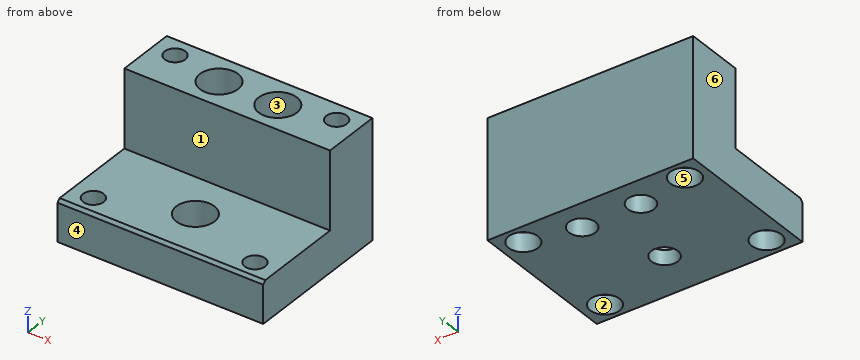
```python
from build123d import *

# Parameters (mm, degrees)
SKIZZE1_W                                            = 140
SKIZZE1_H                                            = 103
BASIS_LINEAR_AUSTRAGEN_DEPTH                         = 40.5
SKIZZE8_W                                            = 53
SKIZZE8_H                                            = 63
SCHNITT_LINEAR_AUSTRAGEN1_DEPTH                      = 155.571989701
BOHRUNG1_D                                           = 18
BOHRUNG1_DEPTH                                       = 90
BOHRUNG1_CBORE_D                                     = 26
BOHRUNG1_CBORE_DEPTH                                 = 18
BOHRUNG2_D                                           = 18
BOHRUNG2_DEPTH                                       = 90
BOHRUNG2_CBORE_D                                     = 26
BOHRUNG2_CBORE_DEPTH                                 = 18
LINEARES_MUSTER1_COUNT                               = 2
LINEARES_MUSTER1_PITCH                               = 40
STIRNSENKUNG_F_R_M8_FLACHKOPFSCHRAUBE_MI_D           = 14
STIRNSENKUNG_F_R_M8_FLACHKOPFSCHRAUBE_MI_CBORE_D     = 20
STIRNSENKUNG_F_R_M8_FLACHKOPFSCHRAUBE_MI_CBORE_DEPTH = 13
SKIZZE11_R                                           = 13
SCHNITT_LINEAR_AUSTRAGEN2_DEPTH                      = 18
FASE1_SIZE                                           = 2


with BuildPart() as part:
    # Skizze1 → Basis-Linear austragen (new, symmetric)
    with BuildSketch(Plane.XY):
        Rectangle(SKIZZE1_W, SKIZZE1_H)
    extrude(amount=BASIS_LINEAR_AUSTRAGEN_DEPTH, both=True)

    # Skizze8 → Schnitt-Linear austragen1 (cut, through all)
    with BuildSketch(Plane.ZY.offset(70)):
        with Locations((14, -20)):
            Rectangle(SKIZZE8_W, SKIZZE8_H)
    extrude(amount=-SCHNITT_LINEAR_AUSTRAGEN1_DEPTH, mode=Mode.SUBTRACT)

    # Bohrung1
    with Locations(Plane.XY.offset(40.5)):
        with Locations((0, -18.5)):
            CounterBoreHole(BOHRUNG1_D / 2, BOHRUNG1_CBORE_D / 2, BOHRUNG1_CBORE_DEPTH, depth=BOHRUNG1_DEPTH)

    # Bohrung2
    with Locations(Plane.XY.offset(40.5)):
        with Locations((20, 31.5)):
            bohrung2 = CounterBoreHole(BOHRUNG2_D / 2, BOHRUNG2_CBORE_D / 2, BOHRUNG2_CBORE_DEPTH, depth=BOHRUNG2_DEPTH)

    # Lineares Muster1: Bohrung2 ×2
    with Locations(*[(-i * LINEARES_MUSTER1_PITCH, 0, 0) for i in range(1, LINEARES_MUSTER1_COUNT)]):
        add(bohrung2, mode=Mode.SUBTRACT)

    # Stirnsenkung für M8 Flachkopfschraube mit Schlitz1 (through all)
    with Locations(Plane(origin=(0, 0, -40.5), x_dir=(-1, 0, 0), z_dir=(0, 0, -1))):
        with Locations((-55, -38.5), (-55, 38.5), (55, 38.5), (55, -38.5)):
            CounterBoreHole(STIRNSENKUNG_F_R_M8_FLACHKOPFSCHRAUBE_MI_D / 2, STIRNSENKUNG_F_R_M8_FLACHKOPFSCHRAUBE_MI_CBORE_D / 2, STIRNSENKUNG_F_R_M8_FLACHKOPFSCHRAUBE_MI_CBORE_DEPTH)

    # Skizze11 → Schnitt-Linear austragen2 (cut)
    with BuildSketch(Plane.XY.offset(-12.5)):
        with Locations((0, -18.5)):
            Circle(SKIZZE11_R)
    extrude(amount=-SCHNITT_LINEAR_AUSTRAGEN2_DEPTH, mode=Mode.SUBTRACT)

    # Fase1
    fase1_edges = [part.edges().sort_by_distance(p)[0] for p in [
        (0, -51.5, -12.5),
    ]]
    chamfer(fase1_edges, length=FASE1_SIZE)


solid = part.part
```
Geometry check sheet. Reference: the model listing, model coordinates, mm. Face numbers are marked on the shaded views. A direction names the side the tool comes from. Round coordinates to 2 decimals unless told otherwise and drop trailing zeros. Loops run counter-clockwise (first coordinate to the right, second up) from the corner with the lowest first, then second, coordinate; pieces in that order, holes last. Notation, with made-up numbers: M 35.25,-10.75 L 41.25,-10.75 A20 ccw 41.25,24.25 Z; hole C -26,51 d3. An arc over 180 degrees is marked long. Return JSON: item names as keys, results as strings. Group by question number.
(1) Scan lines: line 1 along X through (y, z) = (-38, -24); line 2 along X through (y, z) = (43, 4.5); line 3 along X through (y, z) = (35.5, 29). Record each from-to range of solid material in increasing order. Write a range as [from, to].
(2) Go/stop test with flat-tipped pins: pin 1 (10 mm diameter, centred on x = -56.5, y = 43, fed in from -Z); pin 2 (16 mm diameter, centred on x = -55, y = -38.5, fed in from +Z); pin 3 (13 mm diameter, centred on x = -0.5, y = -22.5, fed in from +Z). Record where each tip stops, or that it passes through.
(3) Section check A-A, the plane x = -20. Enter the section's corners in (y, z), and give its area (3 significant figures).
(4) Section check D-D, the plane y = -18.5. Enter the section's corners in (x, z), and give its area (3 significant figures).
(5) Section check C-C, the plane y = -38.5. Enter the section's corners in (x, z).
(6) Section check B-B, the plane z = 10. Enter the section's corners in (x, y).
(7) Mould release check, pull along Y, two halves, no side actions. Record for the marked faces 4, 5 and 6: pulls with the +Y half, pulls with the -Y half, needs draft (parallel to the pull), parting line crosses it, or undercut.
(8) Set-up check for the marked faces 1, 2 and 3: record each of +Z, -Z, +X, -X, +Y, -Y from which the full face is reachable in a straight line by a thin tool's end or side.
Data:
{
 "1": {"line 1": "[-70, -61.98], [-48.02, 48.02], [61.98, 70]", "line 2": "[-70, -60.36], [-49.64, 49.64], [60.36, 70]", "line 3": "[-70, -61.32], [-48.68, -32.37], [-7.63, 7.63], [32.37, 48.68], [61.32, 70]"},
 "2": {"pin 1": "z = -27.5", "pin 2": "z = -12.5", "pin 3": "z = -30.5"},
 "3": {"outline": "M -51.5,-40.5 L 22.5,-40.5 L 22.5,22.5 L 18.5,22.5 L 18.5,40.5 L 11.5,40.5 L 11.5,-12.5 L -49.5,-12.5 L -51.5,-14.5 Z; M 40.5,-40.5 L 51.5,-40.5 L 51.5,40.5 L 44.5,40.5 L 44.5,22.5 L 40.5,22.5 Z", "area": "3,400 mm²"},
 "4": {"outline": "M -70,-40.5 L -9,-40.5 L -9,-30.5 L -13,-30.5 L -13,-12.5 L -70,-12.5 Z; M 9,-40.5 L 70,-40.5 L 70,-12.5 L 13,-12.5 L 13,-30.5 L 9,-30.5 Z", "area": "3,270 mm²"},
 "5": {"outline": "M -70,-40.5 L -65,-40.5 L -65,-27.5 L -62,-27.5 L -62,-12.5 L -70,-12.5 Z; M -48,-27.5 L -45,-27.5 L -45,-40.5 L 45,-40.5 L 45,-27.5 L 48,-27.5 L 48,-12.5 L -48,-12.5 Z; M 62,-27.5 L 65,-27.5 L 65,-40.5 L 70,-40.5 L 70,-12.5 L 62,-12.5 Z"},
 "6": {"outline": "M -70,11.5 L 70,11.5 L 70,51.5 L -70,51.5 Z; hole C -55,38.5 d14; hole C -20,31.5 d18; hole C 20,31.5 d18; hole C 55,38.5 d14"},
 "7": {"face 4": "pulls with the -Y half", "face 5": "undercut", "face 6": "needs draft"},
 "8": {"face 1": "+Z, +X, -X, -Y", "face 2": "-Z", "face 3": "+Z"}
}
